```python
from build123d import *

# Parameters (mm, degrees)
SKETCH_1_W             = 61.5
SKETCH_1_H             = 20
EXTRUDE_1_DEPTH        = 3
EXTRUDE_2_DEPTH        = 3
PATTERN_LINEAR_1_COUNT = 16
PATTERN_LINEAR_1_PITCH = 3.141592654
CUT_EXTRUDE_1_REACH    = 5
SKETCH_3_R             = 1.65
CUT_EXTRUDE_2_REACH    = 5
SKETCH_4_R             = 1.65
CHAMFER_1_SIZE         = 5


with BuildPart() as part:
    # 草圖1 → 填料-伸長1 (new body)
    with BuildSketch(Plane.XY):
        Rectangle(SKETCH_1_W, SKETCH_1_H)
    extrude(amount=EXTRUDE_1_DEPTH)

    # 草圖2 → 填料-伸長2 (add)
    with BuildSketch(Plane.XY.offset(3)):
        Polygon((-29.75, 10), (-28.931066973, 12.25), (-28.088211111, 12.25), (-27.269278084, 10), align=None)
    extrude_2 = extrude(amount=-EXTRUDE_2_DEPTH)

    # 直線複製排列1: 填料-伸長2 ×16
    with Locations(*[(i * PATTERN_LINEAR_1_PITCH, 0, 0) for i in range(1, PATTERN_LINEAR_1_COUNT)]):
        add(extrude_2)

    # 草圖3 → 除料-伸長1 (cut, up to next)
    with BuildSketch(Plane.XY.offset(3), mode=Mode.PRIVATE) as cut_extrude_1_sk1:
        with Locations((-21.75, 6)):
            Circle(SKETCH_3_R)
    cut_extrude_1_tool1 = extrude(cut_extrude_1_sk1.sketch, amount=-CUT_EXTRUDE_1_REACH, mode=Mode.PRIVATE) & part.part
    add(cut_extrude_1_tool1.solids().sort_by_distance((-21.75, 6, 3))[0], mode=Mode.SUBTRACT)
    # 草圖3 → 除料-伸長1 (cut, up to next)
    with BuildSketch(Plane.XY.offset(3), mode=Mode.PRIVATE) as cut_extrude_1_sk2:
        with Locations((-13.75, 6)):
            Circle(SKETCH_3_R)
    cut_extrude_1_tool2 = extrude(cut_extrude_1_sk2.sketch, amount=-CUT_EXTRUDE_1_REACH, mode=Mode.PRIVATE) & part.part
    add(cut_extrude_1_tool2.solids().sort_by_distance((-13.75, 6, 3))[0], mode=Mode.SUBTRACT)
    # 草圖3 → 除料-伸長1 (cut, up to next)
    with BuildSketch(Plane.XY.offset(3), mode=Mode.PRIVATE) as cut_extrude_1_sk3:
        with Locations((-21.75, -6)):
            Circle(SKETCH_3_R)
    cut_extrude_1_tool3 = extrude(cut_extrude_1_sk3.sketch, amount=-CUT_EXTRUDE_1_REACH, mode=Mode.PRIVATE) & part.part
    add(cut_extrude_1_tool3.solids().sort_by_distance((-21.75, -6, 3))[0], mode=Mode.SUBTRACT)
    # 草圖3 → 除料-伸長1 (cut, up to next)
    with BuildSketch(Plane.XY.offset(3), mode=Mode.PRIVATE) as cut_extrude_1_sk4:
        with Locations((-13.75, -6)):
            Circle(SKETCH_3_R)
    cut_extrude_1_tool4 = extrude(cut_extrude_1_sk4.sketch, amount=-CUT_EXTRUDE_1_REACH, mode=Mode.PRIVATE) & part.part
    add(cut_extrude_1_tool4.solids().sort_by_distance((-13.75, -6, 3))[0], mode=Mode.SUBTRACT)

    # 草圖4 → 除料-伸長2 (cut, up to next)
    with BuildSketch(Plane.XY.offset(3), mode=Mode.PRIVATE) as cut_extrude_2_sk1:
        with Locations((23.75, 5)):
            Circle(SKETCH_4_R)
    cut_extrude_2_tool1 = extrude(cut_extrude_2_sk1.sketch, amount=-CUT_EXTRUDE_2_REACH, mode=Mode.PRIVATE) & part.part
    add(cut_extrude_2_tool1.solids().sort_by_distance((23.75, 5, 3))[0], mode=Mode.SUBTRACT)
    # 草圖4 → 除料-伸長2 (cut, up to next)
    with BuildSketch(Plane.XY.offset(3), mode=Mode.PRIVATE) as cut_extrude_2_sk2:
        with Locations((13.75, 5)):
            Circle(SKETCH_4_R)
    cut_extrude_2_tool2 = extrude(cut_extrude_2_sk2.sketch, amount=-CUT_EXTRUDE_2_REACH, mode=Mode.PRIVATE) & part.part
    add(cut_extrude_2_tool2.solids().sort_by_distance((13.75, 5, 3))[0], mode=Mode.SUBTRACT)
    # 草圖4 → 除料-伸長2 (cut, up to next)
    with BuildSketch(Plane.XY.offset(3), mode=Mode.PRIVATE) as cut_extrude_2_sk3:
        with Locations((23.75, -5)):
            Circle(SKETCH_4_R)
    cut_extrude_2_tool3 = extrude(cut_extrude_2_sk3.sketch, amount=-CUT_EXTRUDE_2_REACH, mode=Mode.PRIVATE) & part.part
    add(cut_extrude_2_tool3.solids().sort_by_distance((23.75, -5, 3))[0], mode=Mode.SUBTRACT)
    # 草圖4 → 除料-伸長2 (cut, up to next)
    with BuildSketch(Plane.XY.offset(3), mode=Mode.PRIVATE) as cut_extrude_2_sk4:
        with Locations((13.75, -5)):
            Circle(SKETCH_4_R)
    cut_extrude_2_tool4 = extrude(cut_extrude_2_sk4.sketch, amount=-CUT_EXTRUDE_2_REACH, mode=Mode.PRIVATE) & part.part
    add(cut_extrude_2_tool4.solids().sort_by_distance((13.75, -5, 3))[0], mode=Mode.SUBTRACT)

    # 導角1
    chamfer_1_edges = [part.edges().sort_by_distance(p)[0] for p in [
        (30.75, -10, 1.5),
        (-30.75, -10, 1.5),
    ]]
    chamfer(chamfer_1_edges, length=CHAMFER_1_SIZE)


solid = part.part
```
The model under review builds one solid part; all positions refer to its coordinate system, in mm. A direction names the side the tool comes from. Round coordinates to 2 decimals unless told otherwise and drop trailing zeros. Loops run counter-clockwise (first coordinate to the right, second up) from the corner with the lowest first, then second, coordinate; pieces in that order, holes last. Notation, with made-up numbers: (-14.75, 49.25) -> (16.25, 49.25) arc R23 ccw to (16.25, 83.25) -> close; hole circle Ø2 at (62, 32). An arc over 180 degrees is marked (long way). Answer in a Markdown table with one row per item.
1) Consider section A-A, the plane y = 6. Write out the cut boundary in (x, z), plus the area to 3 significant figures.
Taken from the geometry:
| item | result |
|---|---|
| outline | (-30.75, 0) -> (-23.4, 0) -> (-23.4, 3) -> (-30.75, 3) -> close; (-20.1, 0) -> (-15.4, 0) -> (-15.4, 3) -> (-20.1, 3) -> close; (-12.1, 0) -> (12.44, 0) -> (12.44, 3) -> (-12.1, 3) -> close; (15.06, 0) -> (22.44, 0) -> (22.44, 3) -> (15.06, 3) -> close; (25.06, 0) -> (30.75, 0) -> (30.75, 3) -> (25.06, 3) -> close |
| area | 149 mm² |
2) Draft analysis for pull direction X (two halves, no side actions). For faces 3 (the flat face through (0, 1, 3)), 4 (the flat face through (28.285, -7.465, 1.479)), 5 (the cylindrical face through (22.1, -4.93, 1.52)), state which applies: pulls with the +X half, pulls with the -X half, needs draft (parallel to the pull), parting line crosses it, or undercut.
Taken from the geometry:
| item | result |
|---|---|
| face 3 | needs draft |
| face 4 | pulls with the +X half |
| face 5 | undercut |
3) Consider section C-C, the plane x = 21.5. Write out the cut boundary in (y, z).
Taken from the geometry:
| item | result |
|---|---|
| outline | (-10, 0) -> (10, 0) -> (10, 3) -> (-10, 3) -> close |
4) Wall thickness on line 1 along Y through (x, z) = (13.75, 1.15); line 2 along X through (y, z) = (4.5, 0.5); line 3 along X through (y, z) = (4.75, 2.7): over which ranges is each line inside the solid? List them lowest first.
Taken from the geometry:
| item | result |
|---|---|
| line 1 | y = -10 to -6.65, -3.35 to 3.35, 6.65 to 10 |
| line 2 | x = -30.75 to -22.44, -21.06 to -14.44, -13.06 to 12.18, 15.32 to 22.18, 25.32 to 30.75 |
| line 3 | x = -30.75 to -22.83, -20.67 to -14.83, -12.67 to 12.12, 15.38 to 22.12, 25.38 to 30.75 |
5) Consider section D-D, the plane y = -6. Write out the cut boundary in (x, z).
Taken from the geometry:
| item | result |
|---|---|
| outline | (-29.75, 0) -> (-23.4, 0) -> (-23.4, 3) -> (-29.75, 3) -> close; (-20.1, 0) -> (-15.4, 0) -> (-15.4, 3) -> (-20.1, 3) -> close; (-12.1, 0) -> (12.44, 0) -> (12.44, 3) -> (-12.1, 3) -> close; (15.06, 0) -> (22.44, 0) -> (22.44, 3) -> (15.06, 3) -> close; (25.06, 0) -> (29.75, 0) -> (29.75, 3) -> (25.06, 3) -> close |
6) Tool access review of faces 1 (the cylindrical face through (15.274, 4.368, 1.521)), 2 (the flat face through (-19.92, 11.11, 1.52)): name each direction out of +Z, -Z, +X, -X, +Y, -Y from which nothing blocks a thin tool from reaching the whole face with its end or side.
Taken from the geometry:
| item | result |
|---|---|
| face 1 | +Z, -Z |
| face 2 | +Z, -Z, +Y |
7) Consider section B-B, the plane z = 2.3. Count the separate pieces of the cut face and the enclosed holes in it, plus the area to 3 significant figures.
Taken from the geometry:
| item | result |
|---|---|
| separate pieces | 1 |
| enclosed holes | 8 |
| area | 1,200 mm² |
8) For pin 1 Ø3 at (x, y) = (-21.75, 6) entering from -Z, flat-tipped, find the tip position at first contact; note if it passes through.
Taken from the geometry:
| item | result |
|---|---|
| pin 1 | passes through |
